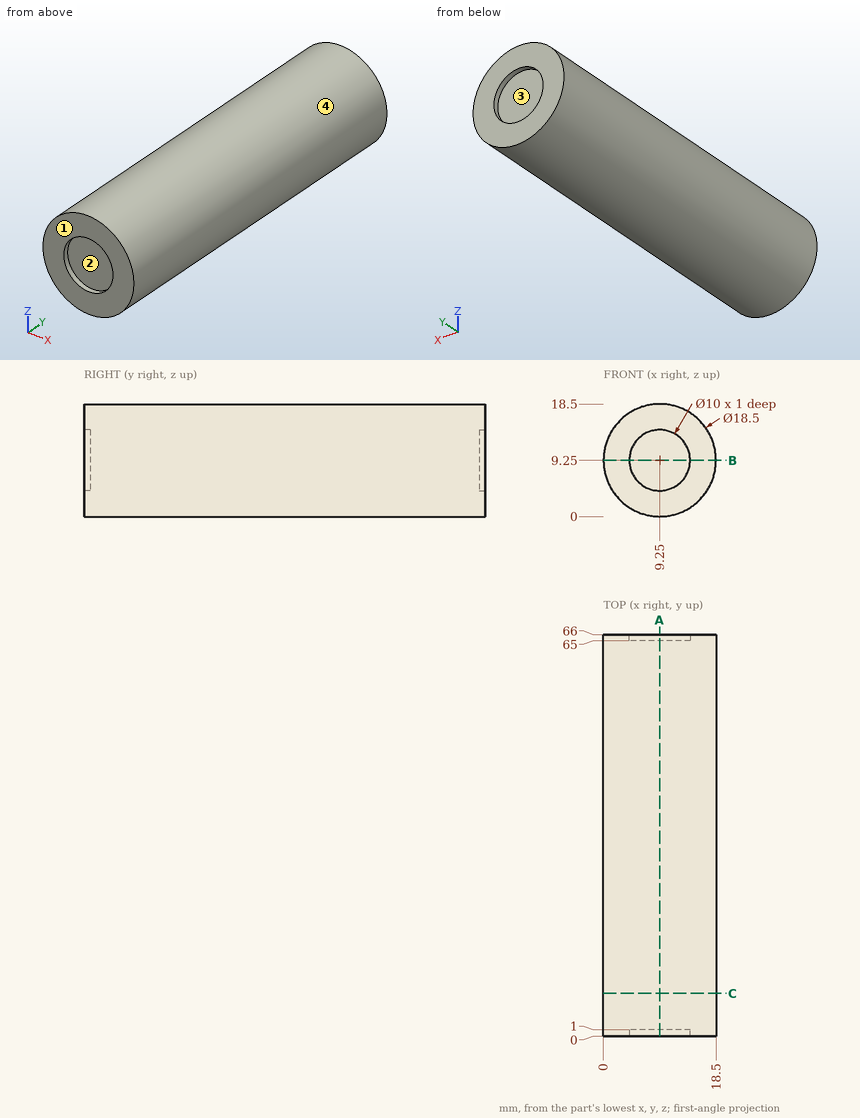
Print and shaded views of the part. All mm, measured from the part's lowest x, y and z. Give positions to 0.01 mm unless a question says otherwise; leave off trailing zeros. Loops run counter-clockwise (first coordinate to the right, second up) from the corner with the lowest first, then second, coordinate; pieces in that order, holes last.
1) Saw through at A-A (x = 9.25). Write the cut outline in (y, z), plus the area to 3 significant figures.
2) Pull direction Z, two halves, no side cores. Call the marked faces 1, 2, 3 and 4: +Z half, -Z half, draft (parallel to the pull), parting line (faces both ways), or undercut.
3) Flat gauge pins, fed straight in: pin 1 Ø6 at (x, z) = (11.5, 10.5) entering from +Y; pin 2 Ø5 at (y, z) = (17.5, 16) entering from -X; pin 3 Ø8 at (x, z) = (9.25, 9.25) entering from -Y; pin 4 Ø3 at (x, z) = (9.5, 11.5) entering from +Y. Where does each tip first touch, or does it go through?
4) Saw through at C-C (y = 7). Write the cut outline in (x, z), plus the area to 3 significant figures.
5) Wall check: line 1 (Z direction, x = 9.25, y = 65.75); line 2 (Y direction, x = 10, z = 11.5); line 3 (X direction, y = 39, z = 6). Give the ranges that are in metal, low to high.
6) Saw through at B-B (z = 9.25). Write the cut outline in (x, y).
Answer block:
1. outline: (0, 0) - (66, 0) - (66, 4.25) - (65, 4.25) - (65, 14.25) - (66, 14.25) - (66, 18.5) - (0, 18.5) - (0, 14.25) - (1, 14.25) - (1, 4.25) - (0, 4.25) - close
1. area: 1,200 mm2
2. face 1: draft
2. face 2: undercut
2. face 3: undercut
2. face 4: parting line
3. pin 1: stops at y = 66
3. pin 2: stops at x = 1.03
3. pin 3: stops at y = 1
3. pin 4: stops at y = 65
4. outline: circle Ø18.5 at (9.25, 9.25)
4. area: 269 mm2
5. line 1: z = 0 to 4.25, 14.25 to 18.5
5. line 2: y = 1 to 65
5. line 3: x = 0.59 to 17.91
6. outline: (0, 0) - (4.25, 0) - (4.25, 1) - (14.25, 1) - (14.25, 0) - (18.5, 0) - (18.5, 66) - (14.25, 66) - (14.25, 65) - (4.25, 65) - (4.25, 66) - (0, 66) - close
